Source: CAD feature listing. Evaluate the final solid. Frame: model axes, mm. Face numbers are marked on the shaded views. Give positions to 0.01 mm unless a question says otherwise; leave off trailing zeros. Answer in a Markdown table with one row per item.
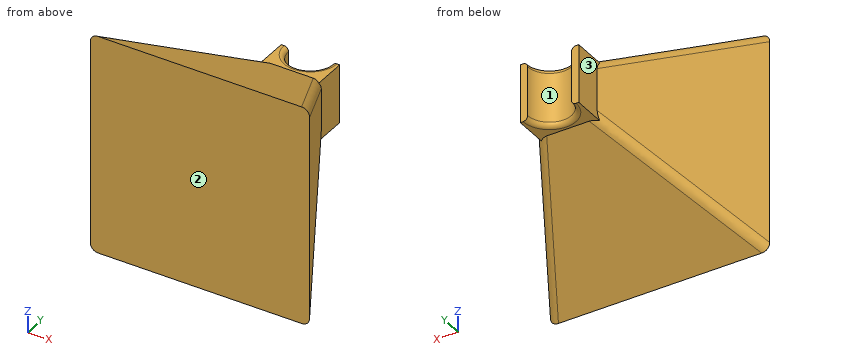
Autodesk Inventor part; units mm, degrees
ref_plane "Work Plane1" through (0, 25.4, 0) normal (0, 1, 0) x (-1, 0, 0)
ref_plane "Work Plane2" through (0, 0, 19.05) normal (0, 0, 1) x (1, 0, 0)
ref_plane "YZ Plane" through (0, 0, 0) normal (1, 0, 0) x (0, 1, 0)
sketch "Sketch1" plane through (0, 0, 0) normal (0, 1, 0) x (-1, 0, 0)
  line L0 (-19.05, 19.05) -> (-19.05, -19.05)
  line L1 (-19.05, -19.05) -> (19.05, -19.05)
  line L2 (19.05, -19.05) -> (19.05, 19.05)
  line L3 (19.05, 19.05) -> (-19.05, 19.05)
  line L4 (-19.05, 19.05) -> (19.05, -19.05) construction
  line L5 (-19.05, -19.05) -> (19.05, 19.05) construction
  point P0 (0, 0)
  dimension "base" = 38.1
ref_plane "Work Plane1" through (0, 25.4, 0) normal (0, 1, 0) x (-1, 0, 0)
sketch "Sketch2" plane through (0, 25.4, 0) normal (0, 1, 0) x (-1, 0, 0)
  line L0 (-5.08, 5.08) -> (-5.08, -5.08)
  line L1 (-5.08, -5.08) -> (5.08, -5.08)
  line L2 (5.08, -5.08) -> (5.08, 5.08)
  line L3 (5.08, 5.08) -> (-5.08, 5.08)
  line L4 (-5.08, 5.08) -> (5.08, -5.08) construction
  line L5 (-5.08, -5.08) -> (5.08, 5.08) construction
  point P0 (0, 0)
  dimension "topOfPyramid" = 10.16
loft "Loft1" add profiles "Sketch1", "Sketch2"
sketch "Sketch3" plane through (0, 0, 0) normal (0, 0, 1) x (1, 0, 0)
  arc A0 (-3.81, 30.48) -> (3.81, 30.48) centre (0, 30.48) ccw
  arc A1 (-5.08, 30.48) -> (5.08, 30.48) centre (0, 30.48) ccw
  line L0 (5.08, 25.4) -> (-5.08, 25.4)
  line L1 (3.81, 30.48) -> (5.08, 30.48)
  line L2 (-3.81, 30.48) -> (-5.08, 30.48)
  line L3 (-5.08, 30.48) -> (-5.08, 25.4)
  line L4 (5.08, 30.48) -> (5.08, 25.4)
  line L5 (19.05, 0) -> (5.08, 25.4)
  line L6 (5.08, 25.4) -> (0, 25.4)
  line L7 (-5.08, 25.4) -> (5.08, 25.4)
  line L8 (-5.08, 25.4) -> (0, 25.4)
  point P0 (0, 0)
  dimension "innerDiamForRope" = 7.62
  dimension "centerForRope" = 5.08
  dimension "outsideDiam" = 10.16
extrude "Extrusion1" add sketch "Sketch3" along normal mid plane 10.16
fillet "Fillet3" radius 1.5875 4 edges at (12.065, 12.7, 12.065) (12.065, 12.7, -12.065) (-12.065, 12.7, 12.065) (-12.065, 12.7, -12.065)
fillet "Fillet5" radius 0.7937 2 edges at (0, 26.67, 5.08) (0, 26.67, -5.08)
ref_plane "Work Plane2" through (0, 0, 19.05) normal (0, 0, 1) x (1, 0, 0)
equation "\"centerForRope\" = 0.5 * outsideDiam"
equation "\"widthOfTop\" = topOfPyramid"
equation "\"d17\" = 0.5 * base"
properties part number "OutdoorSupportForMouseWire"
Q1. Contact query for flat-ended pins moving along their axis: pin 1 Ø3 at (x, y) = (0, 14) entering from -Z (3 decimals); pin 2 Ø4 at (x, z) = (10.5, -11.5) entering from +Y; pin 3 Ø12 at (y, z) = (20, -3) entering from +X. Output: stop coordinate, or through.
Values follow:
| item | result |
|---|---|
| pin 1 | z = -12.175 |
| pin 2 | y = 16.4 |
| pin 3 | x = 11.35 |
Q2. Ray query, probe 1 along X at (y, z) = (5, 15); probe 2 along X at (y, z) = (7, 12); probe 3 along Y at (x, z) = (-16.5, 2). Return the intervals inside material, ascending. Write a range as from..to.
Values follow:
| item | result |
|---|---|
| probe 1 | -16.3..16.3 |
| probe 2 | -15.2..15.2 |
| probe 3 | 0..4.64 |
Q3. Mould query, pull axis X, two halves, no side actions, for the marked faces 1, 2 and 3. Classes: +X half, -X half, draft (parallel to the pull), parting line (faces both ways), or undercut.
Values follow:
| item | result |
|---|---|
| face 1 | undercut |
| face 2 | draft |
| face 3 | -X half |
